Verification items for this drawing (mm, ordinates from the low corner). A direction names the side the tool comes from. Coordinates: 2 decimals unless noted, no trailing zeros. Loops run counter-clockwise (first coordinate to the right, second up) from the corner with the lowest first, then second, coordinate; pieces in that order, holes last. Notation, with made-up numbers: (-7, 40.5) -> (45, 40.5) arc R32 cw to (45, 70.5) -> close; hole circle Ø7 at (0, -18). An arc over 180 degrees is marked (long way). Write item = value, one per line.
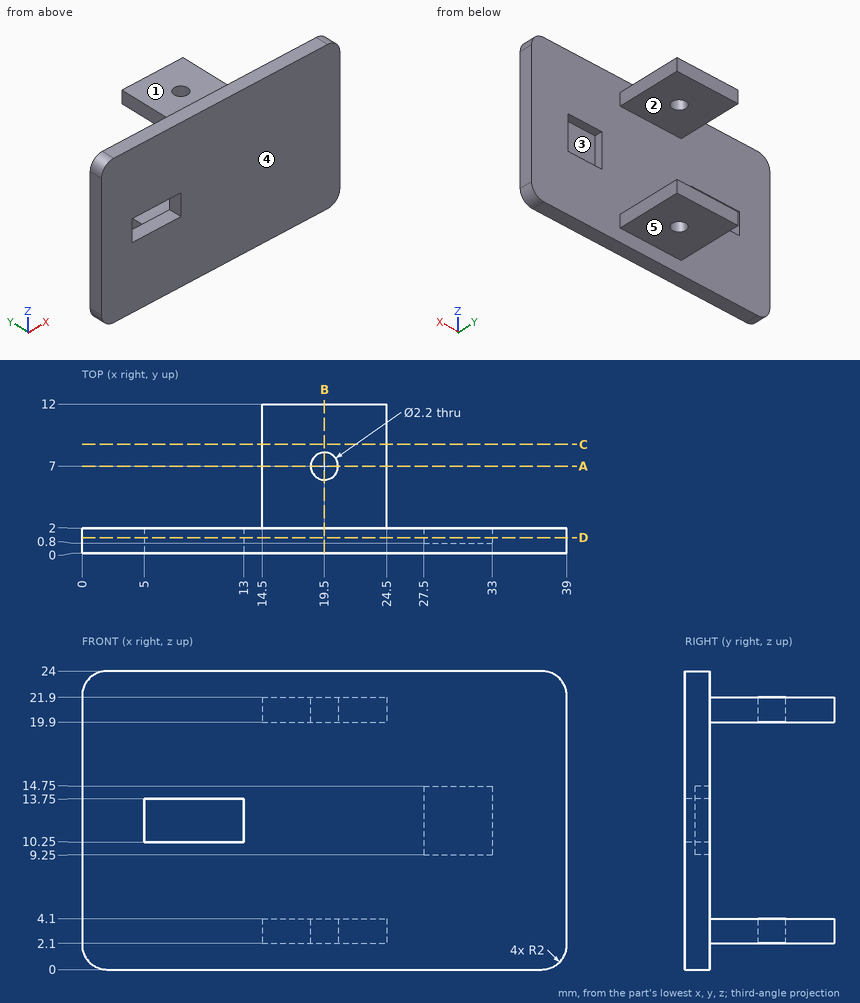
1) Sectioned sample at D-D, the plane y = 1.25. Record the cut outline in (x, z), plus the area to 3 significant figures.
Ans:
outline = (0, 2) arc R2 ccw to (2, 0) -> (37, 0) arc R2 ccw to (39, 2) -> (39, 22) arc R2 ccw to (37, 24) -> (2, 24) arc R2 ccw to (0, 22) -> close; hole (5, 10.25) -> (13, 10.25) -> (13, 13.75) -> (5, 13.75) -> close; hole (27.5, 9.25) -> (33, 9.25) -> (33, 14.75) -> (27.5, 14.75) -> close
area = 874 mm2
2) Tool access check on the marked faces 1 and 2. Record the directions out of +Z, -Z, +X, -X, +Y, -Y that give a thin tool (end or side, any length) a straight path to the whole face; none if there is none.
Ans:
face_1 = +Z, +X, -X, +Y
face_2 = +X, -X, +Y
3) Sectioned sample at C-C, the plane y = 8.75. Record the cut outline in (x, z).
Ans:
outline = (14.5, 2.1) -> (24.5, 2.1) -> (24.5, 4.1) -> (14.5, 4.1) -> close; (14.5, 19.9) -> (24.5, 19.9) -> (24.5, 21.9) -> (14.5, 21.9) -> close
4) Material ranges on line 1 (Z direction, x = 23, y = 8.75); line 2 (Y direction, x = 19.5, z = 21.05); line 3 (Y direction, x = 30, z = 10), recorded low to high.
Ans:
line_1 = 2.1 to 4.1, 19.9 to 21.9
line_2 = 0 to 5.9, 8.1 to 12
line_3 = 0 to 0.8
5) Depth check by flat-ended pin: pin 1 Ø5 at (x, y) = (20.5, 8.5) entering from -Z; pin 2 Ø6 at (x, y) = (22.5, 4) entering from -Z; pin 3 Ø1 at (y, z) = (8.5, 3) entering from +X; pin 4 Ø3 at (x, z) = (33, 3) entering from +Y. Enter the tip coordinate at first touch or a pass-through.
Ans:
pin_1 = 2.1
pin_2 = 0
pin_3 = 24.5
pin_4 = 2
6) Sectioned sample at B-B, the plane x = 19.5. Record the cut outline in (y, z), plus the area to 3 significant figures.
Ans:
outline = (0, 0) -> (2, 0) -> (2, 2.1) -> (5.9, 2.1) -> (5.9, 4.1) -> (2, 4.1) -> (2, 19.9) -> (5.9, 19.9) -> (5.9, 21.9) -> (2, 21.9) -> (2, 24) -> (0, 24) -> close; (8.1, 2.1) -> (12, 2.1) -> (12, 4.1) -> (8.1, 4.1) -> close; (8.1, 19.9) -> (12, 19.9) -> (12, 21.9) -> (8.1, 21.9) -> close
area = 79.2 mm2
7) Sectioned sample at A-A, the plane y = 7. Record the cut outline in (x, z), plus the area to 3 significant figures.
Ans:
outline = (14.5, 2.1) -> (18.4, 2.1) -> (18.4, 4.1) -> (14.5, 4.1) -> close; (14.5, 19.9) -> (18.4, 19.9) -> (18.4, 21.9) -> (14.5, 21.9) -> close; (20.6, 2.1) -> (24.5, 2.1) -> (24.5, 4.1) -> (20.6, 4.1) -> close; (20.6, 19.9) -> (24.5, 19.9) -> (24.5, 21.9) -> (20.6, 21.9) -> close
area = 31.2 mm2
8) Release check for a two-part mould opening along Z. For the marked faces 3, 4 and 5 record: pulls with the +Z half, pulls with the -Z half, needs draft (parallel to the pull), parting line crosses it, or undercut.
Ans:
face_3 = undercut
face_4 = needs draft
face_5 = pulls with the -Z half
